Source: CAD feature listing. Evaluate the final solid. Frame: model axes, mm. Face numbers are marked on the shaded views. A direction names the side the tool comes from. Give positions to 0.01 mm unless a question says otherwise; leave off trailing zeros. Write each loop counter-clockwise with the first axis right and the second up, starting at its lowest first coordinate (ties: lowest second). Pieces come first, ordered by that corner, then holes. Notation, with made-up numbers: (-4.75, 38.25) - (1.25, 38.25) arc R9 cw to (1.25, 51.25) - close; hole circle Ø1 at (35.5, 39.25). An arc over 180 degrees is marked (long way). One line per question, with ' | ' between items. Start each with the question number.
(1) Access query for the marked faces 1 and 2. Directions: +Z, -Z, +X, -X, +Y, -Y. A direction counts if a zero-diameter tool reaches every point of the face in a straight line with its end or side. Return the directions, or none.
(2) Ray query, line 1 (X direction, y = -6, z = 22.5); line 2 (Z direction, x = 18.5, y = -6.5); line 3 (Y direction, x = -9.5, z = 24.75). Return the intervals inside material, ascending. Write a range as [from, to].
(3) Section C-C, the plane y = 0. Return loops of the section in (x, z), plus the area to 3 significant figures.
(4) Section A-A, the plane x = 8. Return loops of the section in (y, z).
(5) Section B-B, the plane z = 20.5. Return loops of the section in (x, y).
(6) Section D-D, the plane y = 3.25. Return loops of the section in (x, z), plus the area to 3 significant figures.
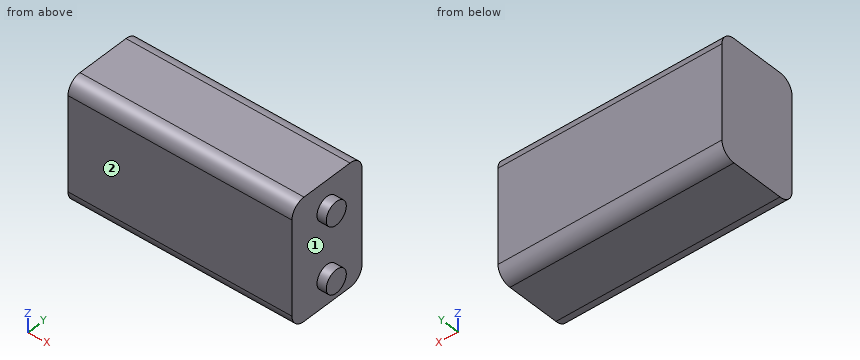
```python
from build123d import *

# Parameters (mm, degrees)
SKETCH_1_W      = 48.5
SKETCH_1_H      = 17.5
EXTRUDE_1_DEPTH = 26.5
FILLET_1_R      = 3
SKETCH_2_R      = 2.5
EXTRUDE_2_DEPTH = 2


with BuildPart() as part:
    # ｽｹｯﾁ1 → ﾎﾞｽ - 押し出し1 (new body)
    with BuildSketch(Plane.XY):
        Rectangle(SKETCH_1_W, SKETCH_1_H)
    extrude(amount=EXTRUDE_1_DEPTH)

    # ﾌｨﾚｯﾄ1
    fillet_1_edges = [part.edges().sort_by_distance(p)[0] for p in [
        (0, -8.75, 26.5),
        (0, -8.75, 0),
        (0, 8.75, 0),
        (0, 8.75, 26.5),
    ]]
    fillet(fillet_1_edges, radius=FILLET_1_R)

    # ｽｹｯﾁ2 → ﾎﾞｽ - 押し出し2 (add)
    with BuildSketch(Plane(origin=(24.25, 0, 0), x_dir=(0, 0, -1), z_dir=(1, 0, 0))):
        with Locations(Location((-20.5, 0, 0), (0, 0, 270))):
            Circle(SKETCH_2_R)
        with Locations(Location((-6, 0, 0), (0, 0, 270))):
            Circle(SKETCH_2_R)
    extrude(amount=EXTRUDE_2_DEPTH)


solid = part.part
```
Check sheet entries:
1) face 1: +X | face 2: +Z, -Z, +X, -X, -Y
2) line 1: [-24.25, 24.25] | line 2: [0.1, 26.4] | line 3: [-8.48, 8.48]
3) outline: (-24.25, 0) - (24.25, 0) - (24.25, 3.5) - (26.25, 3.5) - (26.25, 8.5) - (24.25, 8.5) - (24.25, 18) - (26.25, 18) - (26.25, 23) - (24.25, 23) - (24.25, 26.5) - (-24.25, 26.5) - close | area: 1,310 mm²
4) outline: (-8.75, 3) arc R3 ccw to (-5.75, 0) - (5.75, 0) arc R3 ccw to (8.75, 3) - (8.75, 23.5) arc R3 ccw to (5.75, 26.5) - (-5.75, 26.5) arc R3 ccw to (-8.75, 23.5) - close
5) outline: (-24.25, -8.75) - (24.25, -8.75) - (24.25, -2.5) - (26.25, -2.5) - (26.25, 2.5) - (24.25, 2.5) - (24.25, 8.75) - (-24.25, 8.75) - close
6) outline: (-24.25, 0) - (24.25, 0) - (24.25, 26.5) - (-24.25, 26.5) - close | area: 1,290 mm²
